The model under review builds one solid part; all positions refer to its coordinate system, in mm. Face numbers are marked on the shaded views. A direction names the side the tool comes from. Round coordinates to 2 decimals unless told otherwise and drop trailing zeros. Write each loop counter-clockwise with the first axis right and the second up, starting at its lowest first coordinate (ties: lowest second). Pieces come first, ordered by that corner, then holes.
Item 1: Draft analysis for pull direction Y (two halves, no side actions). For the marked faces 1, 2 and 3, state which applies: +Y half, -Y half, draft (parallel to the pull), parting line (faces both ways), or undercut.
Item 2: Add section C-C (y = 8.5). State how many separate pieces and enclosed holes the cut face has, plus the area to 3 significant figures.
Item 3: Add section A-A (z = -7.75). Give the boundary of the cut face in (x, y).
Item 4: To check wall thickness, follow L1, parallel to X at y = 5.6, z = -18.5; L2, parallel to Z at x = 28, y = 42.55; L3, parallel to Z at x = -17, y = 15.5. State the ranges of each line that lie inside material, in increasing order.
Item 5: Machinability: for the marked faces 4 and 5, which of the approach directions +Z, -Z, +X, -X, +Y, -Y give a long, thin tool a straight path to every point of the face, cutting with its end or side? Answer none if there is none.
Item 6: Add section B-B (z = 27). Give the boundary of the cut face in (x, y).
```python
from build123d import *

# Parameters (mm, degrees)
BOSS_EXTRUDE1_DEPTH      = 30
BOSS_EXTRUDE1_DEPTH_BACK = 30
SKETCH2_W                = 74
SKETCH2_H                = 39
SKETCH2_W_2              = 70
SKETCH2_H_2              = 35
CUT_EXTRUDE1_DEPTH       = 65.171644829
CUT_EXTRUDE1_DEPTH_BACK  = 65.171644829
SKETCH1_R                = 1.25
SKETCH1_R_2              = 2.5
CUT_EXTRUDE2_START       = -37
CUT_EXTRUDE2_DEPTH       = 74
SKETCH4_R                = 1.75
CUT_EXTRUDE3_DEPTH       = 3
CUT_EXTRUDE4_DEPTH       = 61.3158354
CUT_EXTRUDE4_DEPTH_BACK  = 61.3158354
SKETCH5_R                = 1.5
SKETCH5_W                = 3.5
SKETCH5_H                = 19.9


# Read off the part's stored shape, not the designer's step: Cut-Extrude2
with BuildPart() as part:
    # Sketch2 → Boss-Extrude1 (new, two sides: drawn at the far end of the back side and taken through both)
    with BuildSketch(Plane(origin=(0, 0, 0), x_dir=(0, 0, -1), z_dir=(1, 0, 0)).offset(-BOSS_EXTRUDE1_DEPTH_BACK)):
        with Locations((0, 23.5)):
            Rectangle(SKETCH2_W, SKETCH2_H)
        with Locations((0, 23.5)):
            Rectangle(SKETCH2_W_2, SKETCH2_H_2, mode=Mode.SUBTRACT)
    extrude(amount=BOSS_EXTRUDE1_DEPTH + BOSS_EXTRUDE1_DEPTH_BACK)

    # Sketch1 → Cut-Extrude1 (cut, two sides: drawn at the far end of the back side and taken through both)
    with BuildSketch(Plane.XY.offset(-CUT_EXTRUDE1_DEPTH_BACK)):
        with Locations((8.5, 20)):
            Circle(SKETCH1_R)
        with Locations((-8.5, 20)):
            Circle(SKETCH1_R)
        with Locations((0, 10)):
            Circle(SKETCH1_R_2)
    extrude(amount=CUT_EXTRUDE1_DEPTH + CUT_EXTRUDE1_DEPTH_BACK, mode=Mode.SUBTRACT)

    # Cut-Extrude2 outline → Cut-Extrude2 (cut)
    with BuildSketch(Plane.XY.offset(CUT_EXTRUDE2_START)):
        Polygon((-6.223385238, 23), (6.291063493, 23), (0.075182746, 29.257087778), align=None)
        Polygon((-13.493003356, 24.235644043), (-4.153418424, 33.513721677), (-10.100273174, 39.5), (-26.5, 39.5), (-26.5, 37.242640687), align=None)
        Polygon((10.385998459, 39.5), (4.331816644, 33.485688948), (13.507019797, 24.249660484), (26.5, 37.242640687), (26.5, 39.5), align=None)
        Polygon((21.757359313, 7.5), (13.5, 15.757359313), (5.242640687, 7.5), align=None)
        Polygon((26.5, 28.757359313), (17.742640687, 20), (26.5, 11.242640687), align=None)
        Polygon((-13.5, 15.757359313), (-21.757359313, 7.5), (-5.242640687, 7.5), align=None)
        with BuildLine():
            Line((2.432627089, 13.175267776), (6.257359313, 17))
            Line((6.257359313, 17), (-6.257359313, 17))
            Line((-6.257359313, 17), (-2.432627089, 13.175267776))
            ThreePointArc((-2.432627089, 13.175267776), (0, 14), (2.432627089, 13.175267776))
        make_face()
        Polygon((-26.5, 11.242640687), (-17.742640687, 20), (-26.5, 28.757359313), align=None)
        Polygon((1.872544824, 39.5), (-1.642886221, 39.5), (0.103215475, 37.742322846), align=None)
    extrude(amount=CUT_EXTRUDE2_DEPTH, mode=Mode.SUBTRACT)

    # Sketch4 → Cut-Extrude3 (cut)
    with BuildSketch(Plane(origin=(0, 43, 0), x_dir=(1, 0, 0), z_dir=(0, 1, 0))):
        with Locations(Location((-20, 27, 0), (0, 0, 270))):
            Circle(SKETCH4_R)
        with Locations(Location((20, 27, 0), (0, 0, 270))):
            Circle(SKETCH4_R)
        with Locations(Location((20, -27, 0), (0, 0, 270))):
            Circle(SKETCH4_R)
        with Locations(Location((-20, -27, 0), (0, 0, 270))):
            Circle(SKETCH4_R)
    extrude(amount=-CUT_EXTRUDE3_DEPTH, mode=Mode.SUBTRACT)

    # Sketch5 → Cut-Extrude4 (cut, two sides: drawn at the far end of the back side and taken through both)
    with BuildSketch(Plane(origin=(0, 6, 0), x_dir=(1, 0, 0), z_dir=(0, 1, 0)).offset(-CUT_EXTRUDE4_DEPTH_BACK)):
        with Locations(Location((-26.460092097, -18.5, 0), (0, 0, 270))):
            Circle(SKETCH5_R)
        with Locations(Location((-26.460092097, 18.5, 0), (0, 0, 270))):
            Circle(SKETCH5_R)
        with Locations(Location((10.539907903, 18.5, 0), (0, 0, 270))):
            Circle(SKETCH5_R)
        with Locations(Location((10.539907903, -18.5, 0), (0, 0, 270))):
            Circle(SKETCH5_R)
        with Locations(Location((28, -7.75, 0), (0, 0, 270))):
            Circle(SKETCH5_R)
        with Locations(Location((28, 7.75, 0), (0, 0, 270))):
            Circle(SKETCH5_R)
        with Locations((16.25, 0)):
            Rectangle(SKETCH5_W, SKETCH5_H)
    extrude(amount=CUT_EXTRUDE4_DEPTH + CUT_EXTRUDE4_DEPTH_BACK, mode=Mode.SUBTRACT)


solid = part.part
```
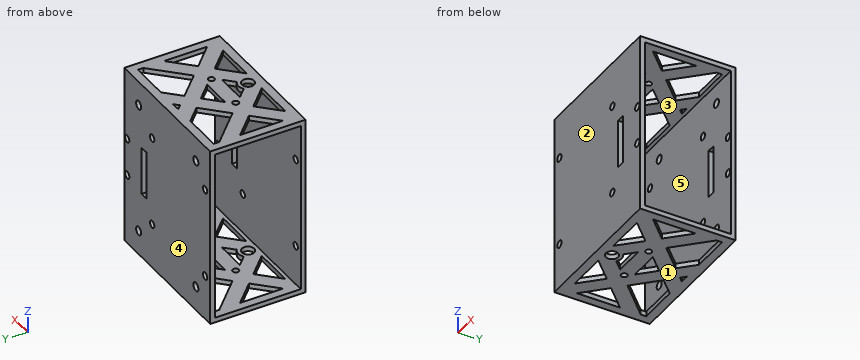
Numbers:
1. face 1: draft
1. face 2: -Y half
1. face 3: undercut
2. separate pieces: 8
2. enclosed holes: 0
2. area: 108 mm2
3. outline: (-30, 4) - (14.5, 4) - (14.5, 6) - (-30, 6) - close; (-30, 41) - (14.5, 41) - (14.5, 43) - (-30, 43) - close; (18, 4) - (26.5, 4) - (26.5, 6) - (18, 6) - close; (18, 41) - (26.5, 41) - (26.5, 43) - (18, 43) - close; (29.5, 4) - (30, 4) - (30, 6) - (29.5, 6) - close; (29.5, 41) - (30, 41) - (30, 43) - (29.5, 43) - close
4. L1: x = -30 to -27.96, -24.96 to 9.04, 12.04 to 30
4. L2: z = -37 to -9.25, -6.25 to 6.25, 9.25 to 37
4. L3: z = -37 to -35, 35 to 37
5. face 4: +Z, -Z, +X, -X, +Y
5. face 5: +X, -X
6. outline: (-30, 4) - (30, 4) - (30, 6) - (-30, 6) - close; (-30, 41) - (-21.75, 41) - (-21.75, 43) - (-30, 43) - close; (-18.25, 41) - (18.25, 41) - (18.25, 43) - (-18.25, 43) - close; (21.75, 41) - (30, 41) - (30, 43) - (21.75, 43) - close
